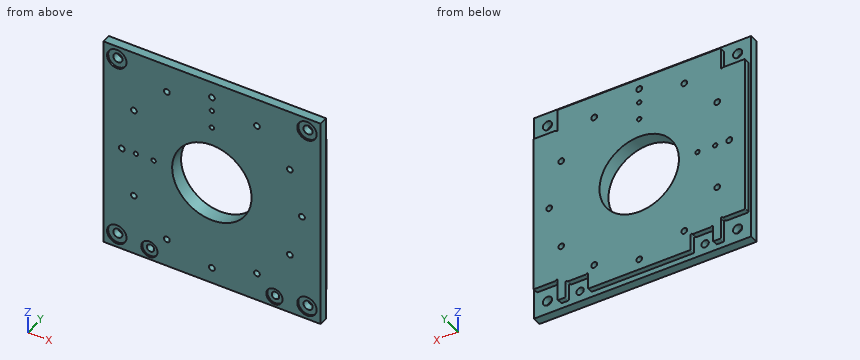
```python
from build123d import *

# Parameters (mm, degrees)
SKETCH_1_W          = 120
SKETCH_1_H          = 120
EXTRUDE_1_DEPTH     = 3
SKETCH_3_W          = 123
SKETCH_3_H          = 120
EXTRUDE_2_DEPTH     = 5
SKETCH_2_R          = 1.65
CUT_EXTRUDE_1_DEPTH = 87.291656607
SKETCH_5_W          = 15.3
SKETCH_5_H          = 15
SKETCH_5_W_2        = 12.6
SKETCH_5_H_2        = 12
CUT_EXTRUDE_2_DEPTH = 3
SKETCH_6_R          = 2.6
SKETCH_6_R_2        = 2.1
CUT_EXTRUDE_3_DEPTH = 87.291656607
SKETCH_7_R          = 5.5
SKETCH_7_R_2        = 4.6
CUT_EXTRUDE_4_DEPTH = 1
SKETCH_8_R          = 22.5
CUT_EXTRUDE_5_DEPTH = 87.291656607
SKETCH_9_R          = 1.25
CUT_EXTRUDE_6_DEPTH = 87.291656607
SKETCH_11_W         = 92.4
SKETCH_11_H         = 3
CUT_EXTRUDE_7_DEPTH = 3
FILLET_1_R          = 0.5
SKETCH_12_R         = 0.5
CUT_EXTRUDE_8_DEPTH = 3
FILLET_2_R          = 1


with BuildPart() as part:
    # 草图1 → 凸台-拉伸1 (new body)
    with BuildSketch(Plane(origin=(0, 0, 0), x_dir=(1, 0, 0), z_dir=(0, 1, 0))):
        Rectangle(SKETCH_1_W, SKETCH_1_H)
    extrude(amount=EXTRUDE_1_DEPTH)

    # 草图3 → 凸台-拉伸2 (add)
    with BuildSketch(Plane.XZ):
        Rectangle(SKETCH_3_W, SKETCH_3_H)
    extrude(amount=EXTRUDE_2_DEPTH)

    # 草图2 → 切除-拉伸1 (cut, through all)
    with BuildSketch(Plane(origin=(0, 3, 0), x_dir=(1, 0, 0), z_dir=(0, 1, 0))):
        with Locations(Location((-51, 0, 0), (0, 0, 270))):
            Circle(SKETCH_2_R)
        with Locations(Location((-44.167295593, -25.5, 0), (0, 0, 270))):
            Circle(SKETCH_2_R)
        with Locations(Location((-25.5, -44.167295593, 0), (0, 0, 270))):
            Circle(SKETCH_2_R)
        with Locations(Location((0, -51, 0), (0, 0, 270))):
            Circle(SKETCH_2_R)
        with Locations(Location((25.5, -44.167295593, 0), (0, 0, 270))):
            Circle(SKETCH_2_R)
        with Locations(Location((44.167295593, -25.5, 0), (0, 0, 270))):
            Circle(SKETCH_2_R)
        with Locations(Location((-25.5, 44.167295593, 0), (0, 0, 270))):
            Circle(SKETCH_2_R)
        with Locations(Location((-44.167295593, 25.5, 0), (0, 0, 270))):
            Circle(SKETCH_2_R)
        with Locations(Location((0, 51, 0), (0, 0, 270))):
            Circle(SKETCH_2_R)
        with Locations(Location((25.5, 44.167295593, 0), (0, 0, 270))):
            Circle(SKETCH_2_R)
        with Locations(Location((44.167295593, 25.5, 0), (0, 0, 270))):
            Circle(SKETCH_2_R)
        with Locations(Location((51, 0, 0), (0, 0, 270))):
            Circle(SKETCH_2_R)
    extrude(amount=-CUT_EXTRUDE_1_DEPTH, mode=Mode.SUBTRACT)

    # 草图5 → 切除-拉伸2 (cut)
    with BuildSketch(Plane(origin=(0, 3, 0), x_dir=(1, 0, 0), z_dir=(0, 1, 0))):
        with Locations((-53.85, 52.5)):
            Rectangle(SKETCH_5_W, SKETCH_5_H)
        with Locations((53.85, 52.5)):
            Rectangle(SKETCH_5_W, SKETCH_5_H)
        with Locations((-35.4, 54)):
            Rectangle(SKETCH_5_W_2, SKETCH_5_H_2)
        with Locations((35.4, 54)):
            Rectangle(SKETCH_5_W_2, SKETCH_5_H_2)
        with Locations((-53.85, -52.5)):
            Rectangle(SKETCH_5_W, SKETCH_5_H)
        with Locations((53.85, -52.5)):
            Rectangle(SKETCH_5_W, SKETCH_5_H)
    extrude(amount=-CUT_EXTRUDE_2_DEPTH, mode=Mode.SUBTRACT)

    # 草图6 → 切除-拉伸3 (cut, through all)
    with BuildSketch(Plane(origin=(0, 3, 0), x_dir=(1, 0, 0), z_dir=(0, 1, 0))):
        with Locations(Location((-53.85, -52.5, 0), (0, 0, 270))):
            Circle(SKETCH_6_R)
        with Locations(Location((53.85, -52.5, 0), (0, 0, 270))):
            Circle(SKETCH_6_R)
        with Locations(Location((-53.85, 52.5, 0), (0, 0, 270))):
            Circle(SKETCH_6_R)
        with Locations(Location((-35.4, 54, 0), (0, 0, 270))):
            Circle(SKETCH_6_R_2)
        with Locations(Location((53.85, 52.5, 0), (0, 0, 270))):
            Circle(SKETCH_6_R)
        with Locations(Location((35.4, 54, 0), (0, 0, 270))):
            Circle(SKETCH_6_R_2)
    extrude(amount=-CUT_EXTRUDE_3_DEPTH, mode=Mode.SUBTRACT)

    # 草图7 → 切除-拉伸4 (cut)
    with BuildSketch(Plane.XZ.offset(5)):
        with Locations(Location((-53.85, 52.5, 0), (0, 0, 270))):
            Circle(SKETCH_7_R)
        with Locations(Location((-53.85, -52.5, 0), (0, 0, 270))):
            Circle(SKETCH_7_R)
        with Locations(Location((-35.4, -54, 0), (0, 0, 270))):
            Circle(SKETCH_7_R_2)
        with Locations(Location((53.85, 52.5, 0), (0, 0, 270))):
            Circle(SKETCH_7_R)
        with Locations(Location((53.85, -52.5, 0), (0, 0, 270))):
            Circle(SKETCH_7_R)
        with Locations(Location((35.4, -54, 0), (0, 0, 270))):
            Circle(SKETCH_7_R_2)
    extrude(amount=-CUT_EXTRUDE_4_DEPTH, mode=Mode.SUBTRACT)

    # 草图8 → 切除-拉伸5 (cut, through all)
    with BuildSketch(Plane(origin=(0, 3, 0), x_dir=(1, 0, 0), z_dir=(0, 1, 0))):
        with Locations(Location((0, 0, 0), (0, 0, 270))):
            Circle(SKETCH_8_R)
    extrude(amount=-CUT_EXTRUDE_5_DEPTH, mode=Mode.SUBTRACT)

    # 草图9 → 切除-拉伸6 (cut, through all)
    with BuildSketch(Plane(origin=(0, 3, 0), x_dir=(1, 0, 0), z_dir=(0, 1, 0))):
        with Locations(Location((0, -43, 0), (0, 0, 270))):
            Circle(SKETCH_9_R)
        with Locations(Location((0, -33, 0), (0, 0, 270))):
            Circle(SKETCH_9_R)
        with Locations(Location((-43, 0, 0), (0, 0, 270))):
            Circle(SKETCH_9_R)
        with Locations(Location((-33, 0, 0), (0, 0, 270))):
            Circle(SKETCH_9_R)
    extrude(amount=-CUT_EXTRUDE_6_DEPTH, mode=Mode.SUBTRACT)

    # 草图11 → 切除-拉伸7 (cut)
    with BuildSketch(Plane(origin=(0, 3, 0), x_dir=(1, 0, 0), z_dir=(0, 1, 0))):
        with Locations((0, -58.5)):
            Rectangle(SKETCH_11_W, SKETCH_11_H)
        with Locations((0, 58.5)):
            Rectangle(SKETCH_11_W, SKETCH_11_H)
    extrude(amount=-CUT_EXTRUDE_7_DEPTH, mode=Mode.SUBTRACT)

    # 圆角1
    fillet_1_edges = [part.edges().sort_by_distance(p)[0] for p in [
        (-60, 1.5, 45),
        (60, 1.5, -45),
        (60, 1.5, 45),
        (-60, 1.5, -45),
        (-46.2, 1.5, 57),
        (46.2, 1.5, 57),
        (-29.1, 1.5, -57),
        (29.1, 1.5, -57),
        (-41.7, 1.5, -57),
        (41.7, 1.5, -57),
        (46.2, 1.5, -57),
        (-46.2, 1.5, -57),
    ]]
    fillet(fillet_1_edges, radius=FILLET_1_R)

    # 草图12 → 切除-拉伸8 (cut)
    with BuildSketch(Plane(origin=(0, 3, 0), x_dir=(1, 0, 0), z_dir=(0, 1, 0))):
        with Locations((-46.7, 45)):
            Circle(SKETCH_12_R)
        with Locations((-41.2, 48)):
            Circle(SKETCH_12_R)
        with Locations((-46.7, -45)):
            Circle(SKETCH_12_R)
        with Locations((41.2, 48)):
            Circle(SKETCH_12_R)
        with Locations((46.7, -45)):
            Circle(SKETCH_12_R)
        with Locations((46.7, 45)):
            Circle(SKETCH_12_R)
        with Locations((-29.6, 48)):
            Circle(SKETCH_12_R)
        with Locations((29.6, 48)):
            Circle(SKETCH_12_R)
    extrude(amount=-CUT_EXTRUDE_8_DEPTH, mode=Mode.SUBTRACT)

    # 圆角2
    fillet_2_edges = [part.edges().sort_by_distance(p)[0] for p in [
        (40.7, 1.5, -48),
        (-30.1, 1.5, -48),
        (-47.2, 1.5, 45),
        (-40.7, 1.5, -48),
        (47.2, 1.5, -45),
        (30.1, 1.5, -48),
        (47.2, 1.5, 45),
        (-47.2, 1.5, -45),
    ]]
    fillet(fillet_2_edges, radius=FILLET_2_R)


solid = part.part
```
Design review of the part built by this model. Coordinates are the model's own, in mm. Give positions to 0.01 mm unless a question says otherwise; leave off trailing zeros. Write each loop counter-clockwise with the first axis right and the second up, starting at its lowest first coordinate (ties: lowest second). Pieces come first, ordered by that corner, then holes.
(1) Clearance check with flat-ended pins moving along their axes: pin 1 Ø2.5 at (x, z) = (0, 51) entering from +Y; pin 2 Ø3.5 at (x, z) = (-55.5, -50) entering from -Y; pin 3 Ø14.5 at (x, z) = (35.4, -54) entering from +Y; pin 4 Ø0.9 at (x, y) = (-8.5, 1.5) entering from -Z. State where each tip first meets the part, or that it passes through.
Checked values:
pin 1: passes through
pin 2: stops at y = -4
pin 3: stops at y = 3
pin 4: stops at z = -57
(2) Add section A-A (z = -25.5). Give the boundary of the cut face in (x, y), and give its area (3 significant figures).
Checked values:
outline: (-61.5, -5) - (-45.82, -5) - (-45.82, 3) - (-60, 3) - (-60, 0) - (-61.5, 0) - close; (-42.52, -5) - (42.52, -5) - (42.52, 3) - (-42.52, 3) - close; (45.82, -5) - (61.5, -5) - (61.5, 0) - (60, 0) - (60, 3) - (45.82, 3) - close
area: 922 mm2
(3) Add section D-D (y = -2.75). Give the number of separate pieces and of enclosed holes in the cut face, and give its area (3 significant figures).
Checked values:
separate pieces: 1
enclosed holes: 23
area: 12,900 mm2
(4) Wall thickness on line 1 along X through (y, z) = (-4, -44); line 2 along X through (y, z) = (-3, 51); line 3 along Z through (x, y) = (-54.5, -1.5): over which ranges is each line inside the solid? List them lowest first.
Checked values:
line 1: x = -61.5 to -27.14, -23.86 to 23.86, 27.14 to 61.5
line 2: x = -61.5 to -55.97, -51.73 to -1.65, 1.65 to 51.73, 55.97 to 61.5
line 3: z = -60 to -55.02, -49.98 to 49.98, 55.02 to 60
(5) Add section B-B (x = -25.5). Give the boundary of the cut face in (y, z).
Checked values:
outline: (-5, -60) - (0, -60) - (0, -57) - (3, -57) - (3, -45.82) - (-5, -45.82) - close; (-5, -42.52) - (3, -42.52) - (3, 42.52) - (-5, 42.52) - close; (-5, 45.82) - (3, 45.82) - (3, 57) - (0, 57) - (0, 60) - (-5, 60) - close
(6) Add section C-C (z = -5). Give the boundary of the cut face in (x, y).
Checked values:
outline: (-61.5, -5) - (-21.94, -5) - (-21.94, 3) - (-60, 3) - (-60, 0) - (-61.5, 0) - close; (21.94, -5) - (61.5, -5) - (61.5, 0) - (60, 0) - (60, 3) - (21.94, 3) - close
